Autodesk Inventor part; units mm, degrees
ref_plane "Work Plane1" through (-9.8149, 0, 0) normal (0, -0.866, -0.5) x (1, 0, 0)
ref_plane "YZ Plane" through (0, 0, 0) normal (1, 0, 0) x (0, 1, 0)
ref_plane "XZ Plane" through (0, 0, 0) normal (0, 1, 0) x (-1, 0, 0)
sketch "Sketch1" plane through (0, 0, 0) normal (1, 0, 0) x (0, 1, 0)
  line L0 (-4.6188, 0) -> (-2.3094, 4)
  line L1 (-2.3094, 4) -> (2.3094, 4)
  line L2 (2.3094, 4) -> (4.6188, 0)
  line L3 (4.6188, 0) -> (2.3094, -4)
  line L4 (2.3094, -4) -> (-2.3094, -4)
  line L5 (-2.3094, -4) -> (-4.6188, 0)
  point P0 (0, 0)
  point P1 (0, 0)
  dimension "d0" = 9.2376
extrude "Body" add sketch "Sketch1" along normal blind 2.7
sketch "Sketch2" plane through (0, 0, 0) normal (0, 0, 1) x (1, 0, 0)
  line L0 (0, 2.3094) -> (0, 4.6188)
  line L1 (0, 4.6188) -> (2.7, 4.6188)
  line L2 (2.7, 2.3094) -> (2.7, 4.6188)
  line L3 (-0.54, 0) -> (3.24, 0)
  line L4 (0.3573, 4.6188) -> (0, 4)
  line L5 (2.3427, 4.6188) -> (2.7, 4)
  dimension "d3" = 30
  dimension "d4" = 30
  dimension "d5" = 8
  dimension "d6" = 8
revolve "Chamfer1" cut sketch "Sketch2" angle 360 about axis through (-10, 0, 0) along (1, 0, 0)
sketch "Sketch3" plane through (2.7, 0, 0) normal (1, 0, 0) x (0, 0, -1)
  arc A0 (-2, -3.4641) -> (2, -3.4641) centre (0, 0) ccw
hole "Thread" at (2.7, 0, 0) direction (-1, 0, 0) diameter 4.134 end through all
chamfer "Chamfer2" distance 0.433 angle 30 1 edges at (2.7, 0, 2.067) measured on face at (2.7, 3.336, -0.083)
chamfer "Chamfer3" distance 0.433 angle 30 1 edges at (0, 0, 2.067) measured on face at (0, 3.336, -0.083)
ref_plane "Work Plane1" through (-9.8149, 0, 0) normal (0, -0.866, -0.5) x (1, 0, 0)
equation "\"d0\" = 1.1547 * SW"
equation "\"d1\" = KOH"
equation "\"d3\" = ANG1"
equation "\"d4\" = ANG2"
equation "\"d5\" = SW0"
equation "\"d6\" = SW01"
equation "\"d8\" = -0.5 * GD1 + 0.5 * NND"
equation "\"d40\" = -0.5 * GD1 + 0.5 * NND"
equation "\"d10\" = -0.5 * GD1 + 0.5 * NND"
equation "\"d41\" = -0.5 * GD1 + 0.5 * NND"
equation "\"ANG1\" = 30deg"
equation "\"ANG2\" = 30deg"
equation "\"NND\" = 5"
equation "\"KOH\" = 2.7"
equation "\"SW\" = 8"
equation "\"SW0\" = SW"
equation "\"SW01\" = SW"
equation "\"GUL\" = 0.541266 * PTC"
equation "\"THREADDIA\" = 5"
equation "\"TOA\" = 30deg"
equation "\"PTC\" = 0.8"
equation "\"E0\" = 1.155 * SW"
equation "\"GAL\" = 0.541266 * PTC"
properties part number "PWTR-0104" material "Steel, Mild"
CAD build for the part. Positions are in the model's coordinates, mm. Coordinates: 2 decimals unless noted, no trailing zeros. Loops run counter-clockwise (first coordinate to the right, second up) from the corner with the lowest first, then second, coordinate; pieces in that order, holes last. Notation, with made-up numbers: (-7.5, 86.5) - (36.5, 86.5) arc R31 cw to (36.5, 112.5) - close; hole circle Ø1 at (8, 40.25). An arc over 180 degrees is marked (long way). Write item = value, one per line. Start each with the question number.
Q1. Pull direction Y, two halves, no side cores. Call faces 1 (the conical face through (0.09, 2.07, -3.6)), 2 (the cylindrical face through (1.33, 1.26, 1.64)), 3 (the conical face through (2.613, -4.15, -0.01)): pulls with the +Y half, pulls with the -Y half, needs draft (parallel to the pull), parting line crosses it, or undercut.
Q2. Cut at A-A, the plane x = 1.3. List the corners of the cut face in (y, z).
Q3. Flat gauge pins, fed straight in: pin 1 Ø1.5 at (x, y) = (1.5, 3.5) entering from +Z; pin 2 Ø2 at (y, z) = (1.5, 1.5) entering from -X. Where does each tip first touch, or does it go through?
Q4. Drill centre lines: L1, parallel to Z at x = 1.05, y = 0; L2, parallel to Y at x = 0.65, z = -1.75; L3, parallel to Y at x = 2.35, z = 1.5. Where is each one in solid material? Low to high.
Computed:
q1.face_1 = pulls with the +Y half
q1.face_2 = undercut
q1.face_3 = pulls with the -Y half
q2.outline = (-4.62, 0) - (-2.31, -4) - (2.31, -4) - (4.62, 0) - (2.31, 4) - (-2.31, 4) - close; hole circle Ø4.13 at (0, 0)
q3.pin_1 = 3.24
q3.pin_2 = 0
q4.L1 = -4 to -2.07, 2.07 to 4
q4.L2 = -3.61 to -1.1, 1.1 to 3.61
q4.L3 = -3.75 to -1.42, 1.42 to 3.75
